```python
from build123d import *

# Parameters (mm, degrees)
SKETCH_1_W          = 76.6
SKETCH_1_H          = 100.8
SKETCH_1_R          = 3.1
EXTRUDE_1_DEPTH     = 8
SKETCH_2_R          = 5.25
CUT_EXTRUDE_1_DEPTH = 6.5
SKETCH_3_R          = 3
EXTRUDE_2_DEPTH     = 1
SKETCH_5_R          = 1.05
CUT_EXTRUDE_2_DEPTH = 64.804780385
SKETCH_6_R          = 2.55
CUT_EXTRUDE_3_DEPTH = 2
SKETCH_7_R          = 1.125
SKETCH_7_R_2        = 4.5
EXTRUDE_3_DEPTH     = 5
FILLET_1_R          = 10
SKETCH_8_R          = 2.5
CUT_EXTRUDE_4_DEPTH = 2.5


with BuildPart() as part:
    # ｽｹｯﾁ1 → ﾎﾞｽ - 押し出し1 (new body)
    with BuildSketch(Plane(origin=(0, 0, 0), x_dir=(1, 0, 0), z_dir=(0, 1, 0))):
        Rectangle(SKETCH_1_W, SKETCH_1_H)
        with Locations(Location((0, 14.4, 0), (0, 0, 270))):
            Circle(SKETCH_1_R, mode=Mode.SUBTRACT)
    extrude(amount=EXTRUDE_1_DEPTH)

    # ｽｹｯﾁ2 → ｶｯﾄ - 押し出し1 (cut)
    with BuildSketch(Plane.XZ):
        with Locations(Location((0, -14.4, 0), (0, 0, 270))):
            Circle(SKETCH_2_R)
    extrude(amount=-CUT_EXTRUDE_1_DEPTH, mode=Mode.SUBTRACT)

    # ｽｹｯﾁ3 → ﾎﾞｽ - 押し出し2 (add)
    with BuildSketch(Plane(origin=(0, 8, 0), x_dir=(1, 0, 0), z_dir=(0, 1, 0))):
        with Locations(Location((0, 28.4, 0), (0, 0, 270))):
            Circle(SKETCH_3_R)
    extrude(amount=EXTRUDE_2_DEPTH)

    # ｽｹｯﾁ5 → ｶｯﾄ - 押し出し2 (cut, through all)
    with BuildSketch(Plane(origin=(0, 8, 0), x_dir=(1, 0, 0), z_dir=(0, 1, 0))):
        with Locations(Location((0, 22.4, 0), (0, 0, 270))):
            Circle(SKETCH_5_R)
        with Locations(Location((8, 22.4, 0), (0, 0, 270))):
            Circle(SKETCH_5_R)
        with Locations(Location((16, 22.4, 0), (0, 0, 270))):
            Circle(SKETCH_5_R)
        with Locations(Location((-8, 22.4, 0), (0, 0, 270))):
            Circle(SKETCH_5_R)
        with Locations(Location((-16, 22.4, 0), (0, 0, 270))):
            Circle(SKETCH_5_R)
        with Locations(Location((-16, 6.4, 0), (0, 0, 90))):
            Circle(SKETCH_5_R)
        with Locations(Location((-8, 6.4, 0), (0, 0, 90))):
            Circle(SKETCH_5_R)
        with Locations(Location((16, 6.4, 0), (0, 0, 90))):
            Circle(SKETCH_5_R)
        with Locations(Location((8, 6.4, 0), (0, 0, 90))):
            Circle(SKETCH_5_R)
        with Locations(Location((0, 6.4, 0), (0, 0, 90))):
            Circle(SKETCH_5_R)
    extrude(amount=-CUT_EXTRUDE_2_DEPTH, mode=Mode.SUBTRACT)

    # ｽｹｯﾁ6 → ｶｯﾄ - 押し出し3 (cut)
    with BuildSketch(Plane(origin=(0, 8, 0), x_dir=(1, 0, 0), z_dir=(0, 1, 0))):
        with Locations(Location((-8, 22.4, 0), (0, 0, 270))):
            Circle(SKETCH_6_R)
        with Locations(Location((-16, 22.4, 0), (0, 0, 270))):
            Circle(SKETCH_6_R)
        with Locations(Location((0, 22.4, 0), (0, 0, 270))):
            Circle(SKETCH_6_R)
        with Locations(Location((8, 22.4, 0), (0, 0, 270))):
            Circle(SKETCH_6_R)
        with Locations(Location((16, 22.4, 0), (0, 0, 270))):
            Circle(SKETCH_6_R)
        with Locations(Location((-8, 6.4, 0), (0, 0, 270))):
            Circle(SKETCH_6_R)
        with Locations(Location((0, 6.4, 0), (0, 0, 270))):
            Circle(SKETCH_6_R)
        with Locations(Location((8, 6.4, 0), (0, 0, 270))):
            Circle(SKETCH_6_R)
        with Locations(Location((16, 6.4, 0), (0, 0, 270))):
            Circle(SKETCH_6_R)
        with Locations(Location((-16, 6.4, 0), (0, 0, 270))):
            Circle(SKETCH_6_R)
    extrude(amount=-CUT_EXTRUDE_3_DEPTH, mode=Mode.SUBTRACT)

    # ｽｹｯﾁ7 → ﾎﾞｽ - 押し出し3 (add)
    with BuildSketch(Plane.XY.offset(50.4)):
        with BuildLine():
            Line((-38.3, 0), (38.3, 0))
            Line((38.3, 0), (38.3, 8))
            Line((38.3, 8), (38.5, 8))
            ThreePointArc((38.5, 8), (48.054475131, 12.20846095), (51.398967948, 22.098532052))
            ThreePointArc((51.398967948, 22.098532052), (47.545941546, 29.995941546), (39.648532052, 33.848967948))
            ThreePointArc((39.648532052, 33.848967948), (39.074832616, 33.887235696), (38.5, 33.9))
            Line((38.5, 33.9), (-38.5, 33.9))
            ThreePointArc((-38.5, 33.9), (-39.074832616, 33.887235696), (-39.648532052, 33.848967948))
            ThreePointArc((-39.648532052, 33.848967948), (-47.545941546, 29.995941546), (-51.398967948, 22.098532052))
            ThreePointArc((-51.398967948, 22.098532052), (-48.054475131, 12.20846095), (-38.5, 8))
            Line((-38.5, 8), (-38.3, 8))
            Line((-38.3, 8), (-38.3, 0))
        make_face()
        with Locations((-38.5, 20.95)):
            Circle(SKETCH_7_R, mode=Mode.SUBTRACT)
        with Locations((-6.5, 20.95)):
            Circle(SKETCH_7_R_2, mode=Mode.SUBTRACT)
        with Locations((38.5, 20.95)):
            Circle(SKETCH_7_R, mode=Mode.SUBTRACT)
        with BuildLine():
            Line((8.75, 24.65), (2.25, 24.65))
            ThreePointArc((2.25, 24.65), (-1.45, 20.95), (2.25, 17.25))
            Line((2.25, 17.25), (8.75, 17.25))
            ThreePointArc((8.75, 17.25), (12.45, 20.95), (8.75, 24.65))
        make_face(mode=Mode.SUBTRACT)
    extrude(amount=EXTRUDE_3_DEPTH)

    # ﾌｨﾚｯﾄ1
    # the kernel refuses this fillet: 10 mm, written as the material it adds along each edge
    with BuildSketch(Plane(origin=(-38.3, 8, 50.4), x_dir=(-0.97737367120093, 0.21151999159232296, 0), z_dir=(0, 0, 1))) as fillet_1_piece_1:
        with BuildLine():
            CenterArc((8.12337112, 9.741069532), FILLET_1_R, 192.211442518, 64.721710974)
            Line((-1.650365592, 7.625869616), (-2.627739263, 7.414349624))
            Line((-2.627739263, 7.414349624), (-0.977373671, -0.211519992))
            Line((-0.977373671, -0.211519992), (0.211519992, -0.977373671))
            ThreePointArc((0.211519992, -0.977373671), (0.406994726, -0.935069673), (5.636406526, -0.974106953))
            Line((5.636406526, -0.974106953), (5.862494216, 0))
        make_face()
    extrude(amount=5)
    with BuildSketch(Plane(origin=(38.3, 8, 50.4), x_dir=(0.9773736712009351, 0.21151999159229984, 0), z_dir=(0, 0, 1))) as fillet_1_piece_2:
        with BuildLine():
            CenterArc((8.12337112, -9.741069532), FILLET_1_R, 103.066846508, 64.721710974)
            Line((-1.650365592, -7.625869616), (-2.627739263, -7.414349624))
            Line((-2.627739263, -7.414349624), (-0.977373671, 0.211519992))
            Line((-0.977373671, 0.211519992), (0.211519992, 0.977373671))
            ThreePointArc((0.211519992, 0.977373671), (0.406994726, 0.935069673), (5.636406526, 0.974106953))
            Line((5.636406526, 0.974106953), (5.862494216, 0))
        make_face()
    extrude(amount=5)

    # ｽｹｯﾁ8 → ｶｯﾄ - 押し出し4 (cut)
    with BuildSketch(Plane.XY.offset(55.4)):
        with Locations((-38.5, 20.95)):
            Circle(SKETCH_8_R)
        with Locations((38.5, 20.95)):
            Circle(SKETCH_8_R)
    extrude(amount=-CUT_EXTRUDE_4_DEPTH, mode=Mode.SUBTRACT)


solid = part.part
```
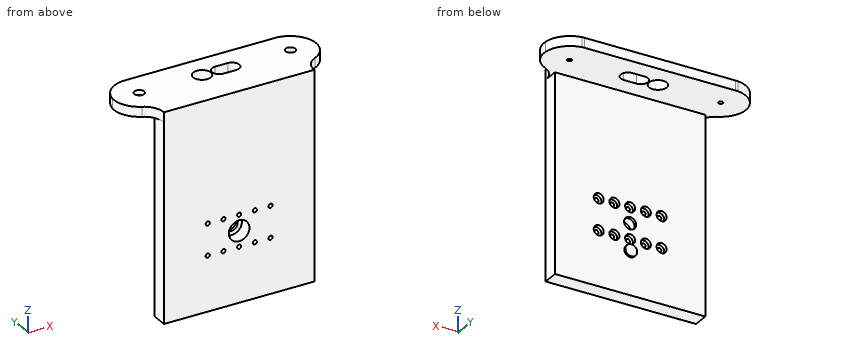
Geometry: final body of the model. Coordinates: model frame, mm. Give positions to 0.01 mm unless a question says otherwise; leave off trailing zeros. Order: outer loops, then holes, each group sorted by start corner. A loop starts at its lowest first (then second) coordinate and runs counter-clockwise, first axis right, second up. Notation, with made-up numbers: M 67,-28 L 97,-28 A23 ccw 97,2 Z; hole C -25,44 d9. An arc over 180 degrees is marked long. Answer as CSV lines item,"result". Start each with the question number.
1) Cut plane C-C (z = 15). Output: boundary loops of the cut face in (x, y), then the cut area to 3 significant figures.
2) Line query: line 1 (X direction, y = 1.85, z = -6.4); line 2 (X direction, y = 7.6, z = -22.4); line 3 (Z direction, x = -17, y = 10). Output: solid intervals per line, ascending. Write a range as from..to.
3) Cut plane D-D (y = 29.5). Output: boundary loops of the cut face in (x, z).
4) First-contact query: P1, Ø5.5, axis at x = 8, z = -7, coming from the +Y side; P2, Ø1.5, axis at x = 1, z = -7.5, coming from the +Y side; P3, Ø12, axis at x = 30.5, y = 18, coming from the -Z side. Flat tips, straight axial feed; report the tip coordinate or a pass-through.
5) Cut plane B-B (x = 26.5). Output: boundary loops of the cut face in (y, z), then the cut area to 3 significant figures.
6) Cut plane A-A (z = -14). Output: boundary loops of the cut face in (x, y).
Findings below:
1,outline,"M -38.3,0 L 38.3,0 L 38.3,8 L -38.3,8 Z"
1,area,"613 mm²"
2,line 1,"x = -38.3..-17.05, -14.95..-9.05, -6.95..-1.05, 1.05..6.95, 9.05..14.95, 17.05..38.3"
2,line 2,"x = -38.3..-18.55, -13.45..-10.55, -5.45..-2.55, 2.55..5.45, 10.55..13.45, 18.55..38.3"
2,line 3,"z = 50.4..55.4"
3,outline,"M -48.02,50.4 L 48.02,50.4 L 48.02,55.4 L -48.02,55.4 Z"
4,P1,"stops at y = 8"
4,P2,"stops at y = 6"
4,P3,"stops at z = 50.4"
5,outline,"M 0,-50.4 L 8,-50.4 L 8,50.4 L 33.9,50.4 L 33.9,55.4 L 0,55.4 Z"
5,area,"976 mm²"
6,outline,"M -38.3,0 L -5.23,0 L -5.23,6.5 L -3.07,6.5 L -3.07,8 L -38.3,8 Z; M 3.07,6.5 L 5.23,6.5 L 5.23,0 L 38.3,0 L 38.3,8 L 3.07,8 Z"
